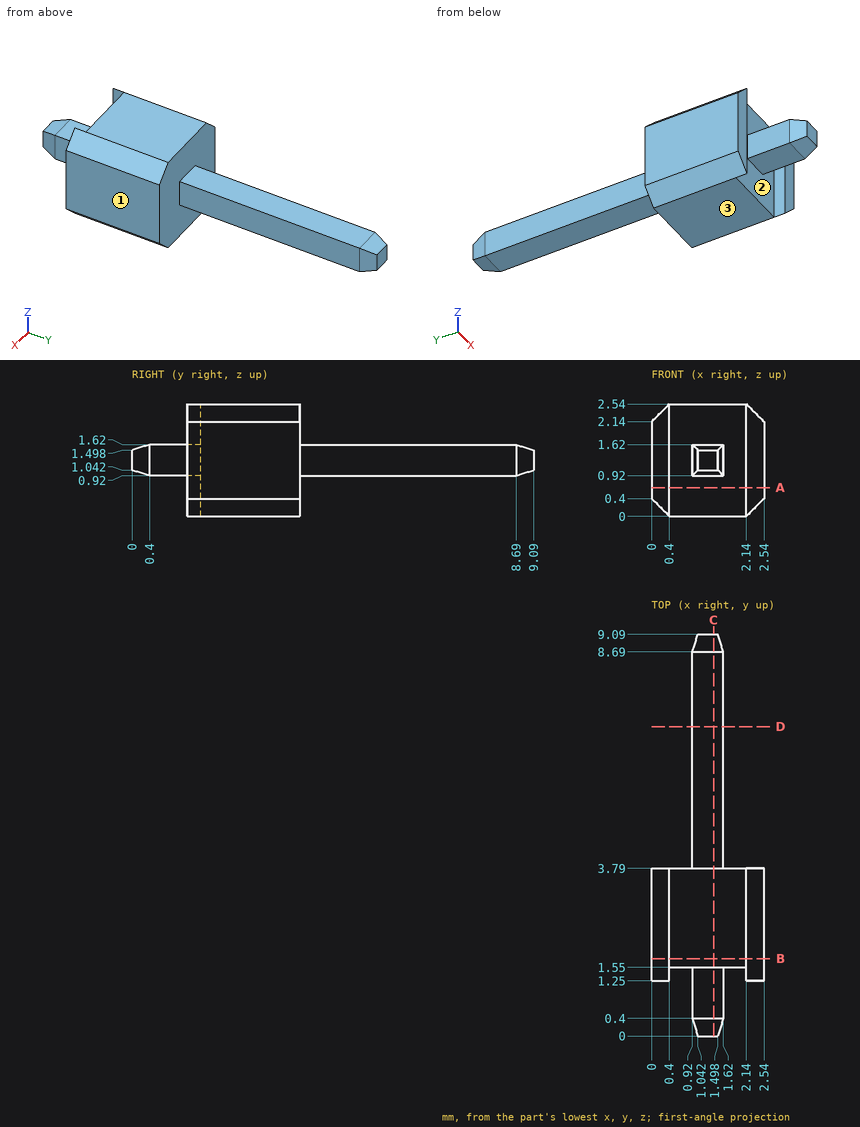
Check sheet for the drawn part. Datum: minimum x, y, z corner. Units: mm. Round coordinates to 2 decimals unless told otherwise and drop trailing zeros. Order: outer loops, then holes, each group sorted by start corner. A loop starts at its lowest first (then second) coordinate and runs counter-clockwise, first axis right, second up.
(1) Go/stop test with flat-tipped pins: P1, Ø0.8, axis at y = 5.5, z = 1.5, coming from the -X side; P2, Ø0.8, axis at x = 1.5, y = 5.5, coming from the -Z side; P3, Ø1.5, axis at x = 0.5, y = 6.5, coming from the +Z side. Record where each tip stops, or that it passes through.
(2) Cross-section at C-C, the plane x = 1.4. Enter the section's corners in (y, z).
(3) Draft check along X on the marked faces 1, 2 and 3. Enter one of: pulls with the +X half, pulls with the -X half, needs draft (parallel to the pull), parting line crosses it, or undercut.
(4) Scan lines: probe 1 along X at (y, z) = (1.5, 1.5); probe 2 along X at (y, z) = (1.5, 2.05); probe 3 along Y at (x, z) = (0.9, 0.3). Record each from-to range of solid material in increasing order.
(5) Cross-section at B-B, the plane y = 1.75. Enter the section's corners in (x, z).
(6) Cross-section at D-D, the plane y = 7. Enter the section's corners in (x, z).
(7) Cross-section at A-A, the plane z = 0.65. Enter the section's corners in (x, y).
Check sheet entries:
1. P1: stops at x = 0.92
1. P2: stops at z = 0.92
1. P3: stops at z = 1.62
2. outline: (0, 1.04) - (0.4, 0.92) - (1.55, 0.92) - (1.55, 0) - (3.79, 0) - (3.79, 0.92) - (8.69, 0.92) - (9.09, 1.04) - (9.09, 1.5) - (8.69, 1.62) - (3.79, 1.62) - (3.79, 2.54) - (1.55, 2.54) - (1.55, 1.62) - (0.4, 1.62) - (0, 1.5) - close
3. face 1: pulls with the +X half
3. face 2: undercut
3. face 3: needs draft
4. probe 1: x = 0 to 0.4, 0.92 to 1.62, 2.14 to 2.54
4. probe 2: x = 0 to 0.4, 2.14 to 2.54
4. probe 3: y = 1.55 to 3.79
5. outline: (0, 0.4) - (0.4, 0) - (2.14, 0) - (2.54, 0.4) - (2.54, 2.14) - (2.14, 2.54) - (0.4, 2.54) - (0, 2.14) - close
6. outline: (0.92, 0.92) - (1.62, 0.92) - (1.62, 1.62) - (0.92, 1.62) - close
7. outline: (0, 1.25) - (0.4, 1.25) - (0.4, 1.55) - (2.14, 1.55) - (2.14, 1.25) - (2.54, 1.25) - (2.54, 3.79) - (0, 3.79) - close
